Source: CAD feature listing. Evaluate the final solid. Frame: model axes, mm. A direction names the side the tool comes from. Give positions to 0.01 mm unless a question says otherwise; leave off trailing zeros. Write each loop counter-clockwise with the first axis right and the second up, starting at its lowest first coordinate (ties: lowest second). Pieces come first, ordered by that corner, then holes. Notation, with made-up numbers: (56, -31.75) -> (60, -31.75) arc R28 cw to (60, -12.75) -> close; hole circle Ø7 at (46.25, 53). An arc over 180 degrees is marked (long way). Use one line per item in the form item = value. Start each with the question number.
(1) Cut plane A-A, the plane x = -103.5. Output: boundary loops of the cut face in (y, z), and give its area (3 significant figures).
(2) First-contact query: P1, Ø8, axis at x = 97, y = 38.5, coming from the -Z side; P2, Ø1.5, axis at y = 23.5, z = 48, coming from the -X side; P3, Ø8, axis at x = 30, z = 8, coming from the +Y side. Flat tips, straight axial feed; report the tip coordinate or a pass-through.
(3) Cut plane D-D, the plane x = -15.5. Output: boundary loops of the cut face in (y, z).
(4) Draft query along Z for faces 4 (the face through (95, 37, 47.5)), 5 (the face through (-123.26, -35, 61.48)), 6 (the face through (-2, 8, 0)). Return one class per face: pulls with the +Z half, pulls with the -Z half, needs draft (parallel to the pull), parting line crosses it, or undercut.
(5) Cut plane C-C, the plane z = 52.5. Output: boundary loops of the cut face in (x, y).
(6) Cut plane B-B, the plane y = 1. Output: boundary loops of the cut face in (x, z).
(7) Set-up query: faces 1 (the face through (90.633, 34.84, 10.923)), 2 (the face through (21.02, -27.5, 1.48)), 3 (the face through (95, 37, 16.5)). Return all of +Z, -Z, +X, -X, +Y, -Y with unobstructed straight access to the full face (end or side cutting, diameter ignored); none if empty.
(8) Material intervals for line 1 along Z through (x, y) = (11, -21.5); line 2 along Y through (x, z) = (67.5, 23); line 3 along Y through (x, z) = (14, 25), sorted ascending. Write a range as from..to.
from build123d import *

# Parameters (mm, degrees)
SKETCH1_R           = 45
SKETCH1_R_2         = 5
SKETCH1_R_3         = 30
BOSS_EXTRUDE1_DEPTH = 3
SKETCH2_W           = 184.390889146
SKETCH2_H           = 63
BOSS_EXTRUDE2_DEPTH = 2
BOSS_EXTRUDE3_START = -3
SKETCH3_R           = 45
SKETCH3_R_2         = 5
SKETCH3_R_3         = 30
BOSS_EXTRUDE3_DEPTH = 3
SKETCH5_R           = 7
SKETCH5_R_2         = 5
BOSS_EXTRUDE4_DEPTH = 2.5
BOSS_EXTRUDE5_START = 2.5
SKETCH7_R           = 7
SKETCH7_R_2         = 5
BOSS_EXTRUDE5_DEPTH = 2.5
SKETCH11_R          = 5
BOSS_EXTRUDE6_DEPTH = 5.5
BOSS_EXTRUDE7_START = 10
SKETCH12_R          = 5
BOSS_EXTRUDE7_DEPTH = 10
SKETCH13_R          = 5
BOSS_EXTRUDE8_DEPTH = 16.5
BOSS_EXTRUDE9_START = 5
BOSS_EXTRUDE9_DEPTH = 5


with BuildPart() as part:
    # Sketch1 → Boss-Extrude1 (new body)
    # profile 1 of 3: a face of its own
    with BuildSketch(Plane.XY):
        with BuildLine():
            Line((88.102445193, 65.890888235), (-90.975875137, 21.948253042))
            ThreePointArc((-90.975875137, 21.948253042), (-52.481172674, 13.65368388), (-35.251817171, -21.755231724))
            ThreePointArc((-35.251817171, -21.755231724), (-42.707811228, -46.563448464), (-62.605044629, -63.150780021))
            Line((-62.605044629, -63.150780021), (107.016332199, 9.158199526))
            ThreePointArc((107.016332199, 9.158199526), (66.791768359, 27.267048462), (88.102445193, 65.890888235))
        make_face()
    # profile 2 of 3: a face of its own
    with BuildSketch(Plane.XY):
        with Locations((-80.251817171, -21.755231724)):
            Circle(SKETCH1_R)
        with Locations((-80.251817171, -21.755231724)):
            Circle(SKETCH1_R_2, mode=Mode.SUBTRACT)
    # profile 3 of 3: a face of its own
    with BuildSketch(Plane.XY):
        with Locations((95.251817171, 36.755231724)):
            Circle(SKETCH1_R_3)
        with Locations((95.251817171, 36.755231724)):
            Circle(SKETCH1_R_2, mode=Mode.SUBTRACT)
    extrude(amount=BOSS_EXTRUDE1_DEPTH)

    # Sketch2 → Boss-Extrude2 (add)
    with BuildSketch(Plane(origin=(-10.246616026, 41.75777759, 0), x_dir=(0.971188550366469, 0.23831239925164718, 0), z_dir=(-0.23831239925164718, 0.971188550366469, 0))):
        with Locations((9.071257122, -31.5)):
            Rectangle(SKETCH2_W, SKETCH2_H)
    extrude(amount=BOSS_EXTRUDE2_DEPTH)

    # Sketch3 → Boss-Extrude3 (add)
    # profile 1 of 3: a face of its own
    with BuildSketch(Plane.XY.offset(63).offset(BOSS_EXTRUDE3_START)):
        with Locations((-80.251817171, -21.755231724)):
            Circle(SKETCH3_R)
        with Locations((-80.251817171, -21.755231724)):
            Circle(SKETCH3_R_2, mode=Mode.SUBTRACT)
    # profile 2 of 3: a face of its own
    with BuildSketch(Plane.XY.offset(63).offset(BOSS_EXTRUDE3_START)):
        with BuildLine():
            ThreePointArc((-35.251817171, -21.755231724), (-42.707811228, -46.563448464), (-62.605044629, -63.150780021))
            Line((-62.605044629, -63.150780021), (107.016332199, 9.158199526))
            ThreePointArc((107.016332199, 9.158199526), (66.791768359, 27.267048462), (88.102445193, 65.890888235))
            Line((88.102445193, 65.890888235), (-90.975875137, 21.948253042))
            ThreePointArc((-90.975875137, 21.948253042), (-52.481172674, 13.65368388), (-35.251817171, -21.755231724))
        make_face()
    # profile 3 of 3: a face of its own
    with BuildSketch(Plane.XY.offset(63).offset(BOSS_EXTRUDE3_START)):
        with Locations((95.251817171, 36.755231724)):
            Circle(SKETCH3_R_3)
        with Locations((95.251817171, 36.755231724)):
            Circle(SKETCH3_R_2, mode=Mode.SUBTRACT)
    extrude(amount=BOSS_EXTRUDE3_DEPTH)

    # Sketch5 → Boss-Extrude4 (add)
    with BuildSketch(Plane.XY.offset(3)):
        with Locations((95.251817171, 36.755231724)):
            Circle(SKETCH5_R)
        with Locations((95.251817171, 36.755231724)):
            Circle(SKETCH5_R_2, mode=Mode.SUBTRACT)
    extrude(amount=BOSS_EXTRUDE4_DEPTH)

    # Sketch7 → Boss-Extrude5 (add)
    with BuildSketch(Plane(origin=(0, 0, 60), x_dir=(-1, 0, 0), z_dir=(0, 0, -1)).offset(BOSS_EXTRUDE5_START)):
        with Locations(Location((-95.251817171, 36.755231724, 0), (0, 0, 180))):
            Circle(SKETCH7_R)
        with Locations(Location((-95.251817171, 36.755231724, 0), (0, 0, 180))):
            Circle(SKETCH7_R_2, mode=Mode.SUBTRACT)
    extrude(amount=-BOSS_EXTRUDE5_DEPTH)

    # Sketch11 → Boss-Extrude6 (add)
    with BuildSketch(Plane(origin=(0, 0, 57.5), x_dir=(-1, 0, 0), z_dir=(0, 0, -1))):
        with Locations(Location((-95.251817171, 36.755231724, 0), (0, 0, 180))):
            Circle(SKETCH11_R)
    extrude(amount=-BOSS_EXTRUDE6_DEPTH)

    # Sketch12 → Boss-Extrude7 (add)
    with BuildSketch(Plane(origin=(0, 0, 57.5), x_dir=(-1, 0, 0), z_dir=(0, 0, -1)).offset(BOSS_EXTRUDE7_START)):
        with Locations(Location((-95.251817171, 36.755231724, 0), (0, 0, 180))):
            Circle(SKETCH12_R)
    extrude(amount=-BOSS_EXTRUDE7_DEPTH)

    # Sketch13 → Boss-Extrude8 (add)
    with BuildSketch(Plane(origin=(0, 0, 0), x_dir=(-1, 0, 0), z_dir=(0, 0, -1))):
        with Locations((-95.251817171, 36.755231724)):
            Circle(SKETCH13_R)
    extrude(amount=-BOSS_EXTRUDE8_DEPTH)

    # Sketch15 → Boss-Extrude9 (add)
    with BuildSketch(Plane(origin=(0, 0, 60), x_dir=(-1, 0, 0), z_dir=(0, 0, -1)).offset(BOSS_EXTRUDE9_START)):
        with BuildLine():
            ThreePointArc((-88.353478337, 35.566568046), (-88.462927218, 35.049074286), (-88.611139115, 34.541322296))
            Line((-88.611139115, 34.541322296), (75.508475702, -20.173867847))
            ThreePointArc((75.508475702, -20.173867847), (75.702840867, -19.679945097), (75.94847072, -19.20940979))
            Line((75.94847072, -19.20940979), (-88.353478337, 35.566568046))
        make_face()
    extrude(amount=-BOSS_EXTRUDE9_DEPTH)


solid = part.part
Geometry says:
q1.outline = (-60.28, 0) -> (16.77, 0) -> (16.77, 3) -> (-60.28, 3) -> close; (-60.28, 60) -> (16.77, 60) -> (16.77, 63) -> (-60.28, 63) -> close
q1.area = 462 mm^2
q2.P1 = 0
q2.P2 = -91.45
q2.P3 = 54.67
q3.outline = (-43.07, 0) -> (42.53, 0) -> (42.53, 63) -> (-43.07, 63) -> (-43.07, 60) -> (-0.17, 60) -> (-0.17, 55) -> (0.94, 55) -> (0.94, 60) -> (40.47, 60) -> (40.47, 3) -> (-43.07, 3) -> close
q4.face_4 = undercut
q4.face_5 = needs draft
q4.face_6 = pulls with the -Z half
q5.outline = (-91.45, 23.89) -> (-90.98, 21.95) -> (88.1, 65.89) -> (87.63, 67.83) -> close; circle Ø10 at (95.25, 36.76)
q6.outline = (-119.07, 0) -> (87.88, 0) -> (87.88, 3) -> (-119.07, 3) -> close; (-119.07, 60) -> (-15.33, 60) -> (-15.33, 55) -> (-12, 55) -> (-12, 60) -> (87.88, 60) -> (87.88, 63) -> (-119.07, 63) -> close
q7.face_1 = none
q7.face_2 = +Z, -Z, +X, -Y
q7.face_3 = +X, +Y, -Y
q8.line_1 = 0..3, 60..63
q8.line_2 = 60.84..62.89
q8.line_3 = 47.71..49.77
